The model under review builds one solid part; all positions refer to its coordinate system, in mm. A direction names the side the tool comes from. Give positions to 0.01 mm unless a question says otherwise; leave off trailing zeros. Order: outer loops, then holes, each group sorted by start corner. A loop starts at its lowest first (then second) coordinate and runs counter-clockwise, first axis right, second up.
```python
from build123d import *

# Parameters (mm, degrees)
SKETCH1_R                = 50
BOSS_EXTRUDE1_DEPTH      = 100
SKETCH6_W                = 25
SKETCH6_H                = 15
BOSS_EXTRUDE3_DEPTH      = 25
FILLET3_R                = 2.5
FILLET4_R                = 10
SKETCH7_R                = 5
CUT_EXTRUDE2_DEPTH       = 25
CIRPATTERN1_COUNT        = 2
FILLET3_OF_CIRPATTERN1_R = 2.5
FILLET4_OF_CIRPATTERN1_R = 10
SKETCH9_W                = 25
SKETCH9_H                = 25
BOSS_EXTRUDE4_DEPTH      = 15
BOSS_EXTRUDE4_DEPTH_BACK = 15
FILLET5_R                = 2.5
FILLET6_R                = 10
SKETCH10_R               = 5
BOSS_EXTRUDE5_DEPTH      = 32.5
BOSS_EXTRUDE5_DEPTH_BACK = 32.5


with BuildPart() as part:
    # Sketch1 → Boss-Extrude1 (new body)
    with BuildSketch(Plane(origin=(0, 0, 0), x_dir=(1, 0, 0), z_dir=(0, 1, 0))):
        Circle(SKETCH1_R)
    extrude(amount=BOSS_EXTRUDE1_DEPTH)

    # Sketch6 → Boss-Extrude3 (add)
    with BuildSketch(Plane(origin=(0, 100, 0), x_dir=(1, 0, 0), z_dir=(0, 1, 0))):
        with Locations((0, -25)):
            Rectangle(SKETCH6_W, SKETCH6_H)
    boss_extrude3 = extrude(amount=BOSS_EXTRUDE3_DEPTH)

    # Fillet3
    fillet3_edges = [part.edges().sort_by_distance(p)[0] for p in [
        (12.5, 100, 25),
        (0, 100, 17.5),
        (-12.5, 100, 25),
        (0, 100, 32.5),
    ]]
    fillet(fillet3_edges, radius=FILLET3_R)

    # Fillet4
    fillet4_edges = [part.edges().sort_by_distance(p)[0] for p in [
        (12.5, 125, 25),
        (-12.5, 125, 25),
    ]]
    fillet(fillet4_edges, radius=FILLET4_R)

    # Sketch7 → Cut-Extrude2 (cut)
    with BuildSketch(Plane.XY.offset(32.5)):
        with Locations((0, 117.5)):
            Circle(SKETCH7_R)
    cut_extrude2 = extrude(amount=-CUT_EXTRUDE2_DEPTH, mode=Mode.SUBTRACT)

    # CirPattern1: Boss-Extrude3, Cut-Extrude2 ×2 about axis
    cirpattern1_axis = Axis((0, 0, 0), (0, 1, 0))
    for i in range(1, CIRPATTERN1_COUNT):
        add(boss_extrude3.rotate(cirpattern1_axis, i * 360 / CIRPATTERN1_COUNT))
        add(cut_extrude2.rotate(cirpattern1_axis, i * 360 / CIRPATTERN1_COUNT), mode=Mode.SUBTRACT)

    # Fillet3 of CirPattern1
    fillet3_of_cirpattern1_edges = [part.edges().sort_by_distance(p)[0] for p in [
        (-12.5, 100, -25),
        (0, 100, -17.5),
        (12.5, 100, -25),
        (0, 100, -32.5),
    ]]
    fillet(fillet3_of_cirpattern1_edges, radius=FILLET3_OF_CIRPATTERN1_R)

    # Fillet4 of CirPattern1
    fillet4_of_cirpattern1_edges = [part.edges().sort_by_distance(p)[0] for p in [
        (-12.5, 125, -25),
        (12.5, 125, -25),
    ]]
    fillet(fillet4_of_cirpattern1_edges, radius=FILLET4_OF_CIRPATTERN1_R)

    # Sketch9 → Boss-Extrude4 (add, two sides)
    with BuildSketch(Plane(origin=(0, 0, 0), x_dir=(0, 0, -1), z_dir=(1, 0, 0))) as boss_extrude4_sk:
        with Locations((0, -12.5)):
            Rectangle(SKETCH9_W, SKETCH9_H)
    extrude(amount=BOSS_EXTRUDE4_DEPTH)
    extrude(boss_extrude4_sk.sketch, amount=-BOSS_EXTRUDE4_DEPTH_BACK)

    # Fillet5
    fillet5_edges = [part.edges().sort_by_distance(p)[0] for p in [
        (0, 0, 12.5),
        (-15, 0, 0),
        (0, 0, -12.5),
        (15, 0, 0),
    ]]
    fillet(fillet5_edges, radius=FILLET5_R)

    # Fillet6
    fillet6_edges = [part.edges().sort_by_distance(p)[0] for p in [
        (0, -25, 12.5),
        (0, -25, -12.5),
    ]]
    fillet(fillet6_edges, radius=FILLET6_R)

    # Sketch10 → Boss-Extrude5 (add, two sides)
    with BuildSketch(Plane(origin=(0, 0, 0), x_dir=(0, 0, -1), z_dir=(1, 0, 0))) as boss_extrude5_sk:
        with Locations((0, -17.5)):
            Circle(SKETCH10_R)
    extrude(amount=BOSS_EXTRUDE5_DEPTH)
    extrude(boss_extrude5_sk.sketch, amount=-BOSS_EXTRUDE5_DEPTH_BACK)


solid = part.part
```
1. Insertion check: pin 1 (2 mm diameter, centred on x = 30, z = 0, fed in from -Y); pin 2 (11 mm diameter, centred on y = -10, z = 0, fed in from -X); pin 3 (6 mm diameter, centred on y = 106.5, z = -28, fed in from +X). Each pin has a flat end and moves straight along its axis. Give the tip position at first contact, or say it passes through.
2. To check wall thickness, follow line 1 (Y direction, x = 0, z = 27); line 2 (Y direction, x = 20, z = 6.5); line 3 (X direction, y = 117, z = -22). State the ranges of each line that lie inside material, in increasing order.
3. For faces 1 (the flat face through (32.5, -17, 0)), 2 (the flat face through (-1, 100, -1)), 3 (the flat face through (0, -9, 12.5)), list the 3-axis set-ups (+Z, -Z, +X, -X, +Y, -Y) from which the entire face can be reached by the end or side of a thin tool; tool diameter is ignored.
4. Draft analysis for pull direction Z (two halves, no side actions). For faces 4 (the flat face through (0, 111, 17.5)), 5 (the flat face through (12.5, 109, 25)), 6 (the flat face through (0, -9, -12.5)), state which applies: pulls with the +Z half, pulls with the -Z half, needs draft (parallel to the pull), parting line crosses it, or undercut.
5. Take a section at C-C (y = 117.5). Write out the cut boundary in (x, z), and give its area (3 significant figures).
6. Take a section at A-A (x = 0). Count the separate pieces of the cut face and the enclosed holes in it, and give its area (3 significant figures).
7. Take a section at D-D (z = 19.5). Write out the cut boundary in (x, y).
8. Take a section at B-B (z = 0). Write out the cut boundary in (x, y).
Answer:
1. pin 1: stops at y = -22.5
1. pin 2: stops at x = -32.5
1. pin 3: stops at x = 12.5
2. line 1: y = 0 to 112.5, 122.5 to 125
2. line 2: y = 0 to 100
2. line 3: x = -12.3 to -4.97, 4.97 to 12.3
3. face 1: +Z, -Z, +X, -Y
3. face 2: +Y
3. face 3: +Z, +X, -X, -Y
4. face 4: undercut
4. face 5: needs draft
4. face 6: pulls with the -Z half
5. outline: (-12.18, -32.5) - (-5, -32.5) - (-5, -17.5) - (-12.18, -17.5) - close; (-12.18, 17.5) - (-5, 17.5) - (-5, 32.5) - (-12.18, 32.5) - close; (5, -32.5) - (12.18, -32.5) - (12.18, -17.5) - (5, -17.5) - close; (5, 17.5) - (12.18, 17.5) - (12.18, 32.5) - (5, 32.5) - close
5. area: 431 mm2
6. separate pieces: 3
6. enclosed holes: 0
6. area: 11,000 mm2
7. outline: (-46.04, 0) - (46.04, 0) - (46.04, 100) - (15, 100) arc R2.5 cw to (12.5, 102.5) - (12.5, 115) arc R10 ccw to (2.5, 125) - (-2.5, 125) arc R10 ccw to (-12.5, 115) - (-12.5, 102.5) arc R2.5 cw to (-15, 100) - (-46.04, 100) - close; hole circle Ø10 at (0, 117.5)
8. outline: (-50, 0) - (-17.5, 0) arc R2.5 cw to (-15, -2.5) - (-15, -12.5) - (-32.5, -12.5) - (-32.5, -22.5) - (-15, -22.5) - (-15, -25) - (15, -25) - (15, -22.5) - (32.5, -22.5) - (32.5, -12.5) - (15, -12.5) - (15, -2.5) arc R2.5 cw to (17.5, 0) - (50, 0) - (50, 100) - (-50, 100) - close
